Check sheet for the drawn part. Datum: minimum x, y, z corner. Units: mm. Round coordinates to 2 decimals unless told otherwise and drop trailing zeros. Write each loop counter-clockwise with the first axis right and the second up, starting at its lowest first coordinate (ties: lowest second). Pieces come first, ordered by that corner, then holes. Notation, with made-up numbers: (-38, 37.5) -> (-4, 37.5) arc R32 ccw to (-4, 64.5) -> close; hole circle Ø11 at (86, -7). An arc over 180 degrees is marked (long way). One line per item, written item: value.
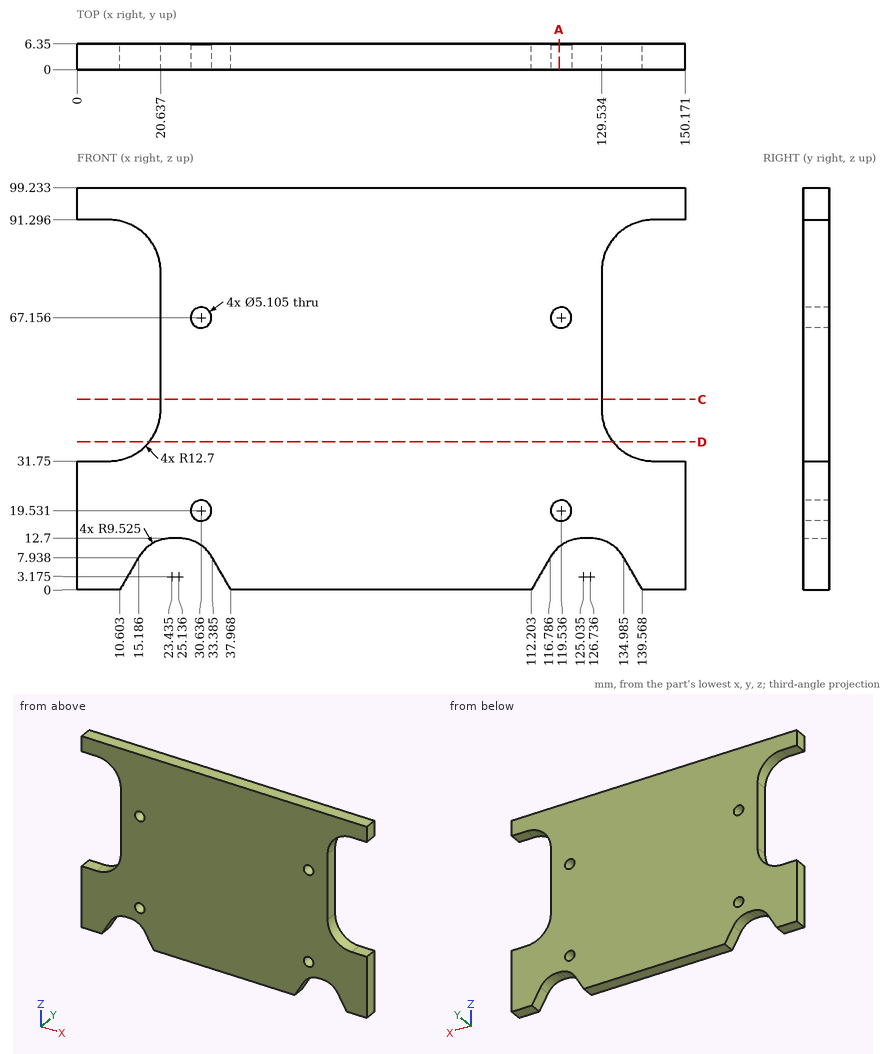
Item 1: Thickness scan on line 1 (X direction, y = 0.75, z = 69) (1 decimal); line 2 (X direction, y = 4.75, z = 7.5) (1 decimal); line 3 (Z direction, x = 131.5, y = 2.5) (1 decimal). Record the ranges inside material, lowest first.
Answer:
line 1: x = 20.6 to 28.9, 32.4 to 117.8, 121.3 to 129.5
line 2: x = 0 to 14.9, 33.6 to 116.5, 135.2 to 150.2
line 3: z = 11.4 to 37.7, 85.4 to 99.2
Item 2: Sectioned sample at A-A on x = 119. Count the separate pieces of the cut face and the enclosed holes in it, and give its area (3 significant figures).
Answer:
separate pieces: 3
enclosed holes: 0
area: 500 mm^2
Item 3: Sectioned sample at D-D on z = 36.5. Enter the section's corners in (x, y), and give its area (3 significant figures).
Answer:
outline: (17.84, 0) -> (132.33, 0) -> (132.33, 6.35) -> (17.84, 6.35) -> close
area: 727 mm^2
Item 4: Depth check by flat-ended pin: P1, Ø6.5, axis at x = 119.54, z = 19.53, coming from the -Y side; P2, Ø0.5, axis at x = 24, y = 4.5, coming from the -Z side; P3, Ø1.9, axis at y = 3.5, z = 55.5, coming from the +X side; P4, Ø3, axis at y = 4.5, z = 84, coming from the +X side (1 decimal). Enter the tip coordinate at first touch or a pass-through.
Answer:
P1: stops at y = 0
P2: stops at z = 12.7
P3: stops at x = 129.53
P4: stops at x = 131.6
Item 5: Sectioned sample at C-C on z = 47. Enter the section's corners in (x, y).
Answer:
outline: (20.64, 0) -> (129.53, 0) -> (129.53, 6.35) -> (20.64, 6.35) -> close
